Verification items for the finished model (mm, model axes). Face numbers are marked on the shaded views. A direction names the side the tool comes from. Round coordinates to 2 decimals unless told otherwise and drop trailing zeros. Loops run counter-clockwise (first coordinate to the right, second up) from the corner with the lowest first, then second, coordinate; pieces in that order, holes last. Notation, with made-up numbers: (-37.5, 6) - (-4.5, 6) arc R24 ccw to (-4.5, 34) - close; hole circle Ø10 at (50.5, 77.25). An arc over 180 degrees is marked (long way). Use a Markdown table: item, result. Add a question column.
```python
from build123d import *

# Parameters (mm, degrees)
F0_R           = 5.5
F1_DEPTH       = 60
F4_DEPTH       = 26
F4_DEPTH_BACK  = 26
F5_R           = 4
F6_DEPTH       = 5
F7_R           = 4.25
F8_DEPTH       = 15
F9_R           = 11
F10_DEPTH      = 25
F10_DEPTH_BACK = 25


# Not quite as in the source:
# - a feature names something its author has since deleted; it is built from what else it names


with BuildPart() as f1:
    # F0 (on Front) → F1 (new body)
    with BuildSketch(Plane.XZ):
        with BuildLine():
            ThreePointArc((-0.0872969156, -53.4805140133), (-11.9999962709, -41.4659778258), (-0.0575900904, -29.4809696761))
            Line((-0.0575900904, -29.4809696761), (-5.4639e-06, 17.0404876904))
            Line((-5.4639e-06, 17.0404876904), (-70.0428405992, 17.0404876904))
            Line((-70.0428405992, 17.0404876904), (-70.0428405992, 7.0404876904))
            Line((-70.0428405992, 7.0404876904), (-20.0428405992, 7.0404876904))
            Line((-20.0428405992, 7.0404876904), (-20.6929361639, -127.9595123096))
            Line((-20.6929361639, -127.9595123096), (-70.6929361639, -127.9595123096))
            Line((-70.6929361639, -127.9595123096), (-70.6929361639, -137.9595123096))
            Line((-70.6929361639, -137.9595123096), (-0.1918656855, -137.9595123096))
            Line((-0.1918656855, -137.9595123096), (-0.1862936956, -133.4580141387))
            ThreePointArc((-0.1862936956, -133.4580141387), (-11.9988136294, -121.4446249335), (-0.1565894029, -109.4605157571))
            Line((-0.1565894029, -109.4605157571), (-0.0872969156, -53.4805140133))
        make_face()
        with Locations((-5.947382655, -81.4808309078)):
            Circle(F0_R, mode=Mode.SUBTRACT)
    extrude(amount=F1_DEPTH)


with BuildPart() as f1_1:
    # F2: moved
    add(f1.part.moved(Location((0, 30, 0))))

    # F3 (on Front) → F4 (cut, two sides)
    with BuildSketch(Plane.XZ) as f4_sk:
        with BuildLine():
            ThreePointArc((0, -55.5154254436), (-14, -41.5154254436), (0, -27.5154254436))
            Line((0, -27.5154254436), (0, -26.5154254436))
            ThreePointArc((0, -26.5154254436), (-15, -41.5154254436), (0, -56.5154254436))
            Line((0, -56.5154254436), (0, -55.5154254436))
        make_face()
        with BuildLine():
            Line((0, -107.5154236555), (0, -106.5154236555))
            ThreePointArc((0, -106.5154236555), (-15, -121.5154236555), (0, -136.5154236555))
            Line((0, -136.5154236555), (0, -135.5154236555))
            ThreePointArc((0, -135.5154236555), (-14, -121.5154236555), (0, -107.5154236555))
        make_face()
    extrude(amount=F4_DEPTH, mode=Mode.SUBTRACT)
    extrude(f4_sk.sketch, amount=-F4_DEPTH_BACK, mode=Mode.SUBTRACT)

    # F5 (on face) → F6 (cut)
    with BuildSketch(Plane.XY.offset(-127.9595123096)):
        with Locations((-40.0428405992, -20)):
            Circle(F5_R)
        with Locations((-40.0428405992, 20)):
            Circle(F5_R)
    extrude(amount=-F6_DEPTH, mode=Mode.SUBTRACT)

    # F7 (on face) → F8 (cut)
    with BuildSketch(Plane.XY.offset(17.0404876904)):
        with Locations((-40.0428405992, 20)):
            Circle(F7_R)
        with Locations((-40.2286797762, -20)):
            Circle(F7_R)
    extrude(amount=-F8_DEPTH, mode=Mode.SUBTRACT)

    # F9 (on face) → F10 (cut, two sides)
    with BuildSketch(Plane.XY.offset(17.0404876904)) as f10_sk:
        with Locations((-40.1357601877, 0)):
            Circle(F9_R)
    extrude(amount=-F10_DEPTH, mode=Mode.SUBTRACT)
    extrude(f10_sk.sketch, amount=F10_DEPTH_BACK, mode=Mode.SUBTRACT)


solid = f1_1.part
```
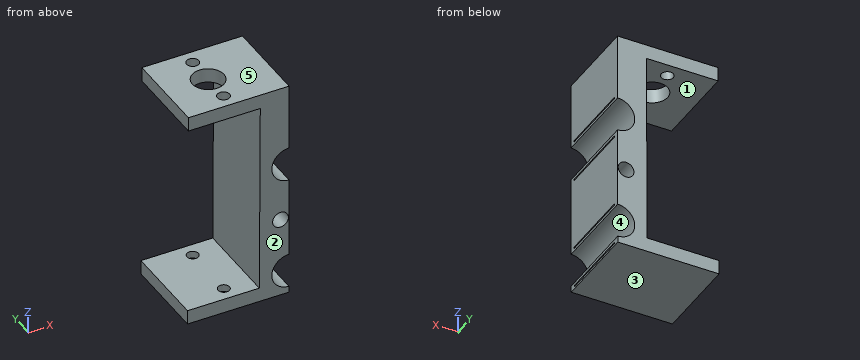
Q1. Section check B-B on x = -57.5. Record the cut outline in (y, z).
Q2. Section check D-D on y = 9. Record the cut outline in (x, z).
Q3. Go/stop test with flat-tipped pins: pin 1 Ø4 at (x, y) = (-38.5, -20.5) entering from +Z; pin 2 Ø8 at (y, z) = (-15, -82.5) entering from -X; pin 3 Ø6.5 at (x, y) = (-42, 19) entering from +Z; pin 4 Ø2 at (y, z) = (-8, -110) entering from -X. Record where each tip stops, or that it passes through.
Q4. Set-up check for the marked faces 1 and 2: record each of +Z, -Z, +X, -X, +Y, -Y from which the full face is reachable in a straight line by a thin tool's end or side.
Q5. Thickness scan on line 1 along Z through (x, y) = (-21, -18.5); line 2 along X through (y, z) = (24.5, -43); line 3 along X through (y, z) = (-13.5, -82). Record the ranges inside material, lowest first.
Q6. Release check for a two-part mould opening along Z. For the marked faces 3, 4 and 5 record: +Z half, -Z half, draft (parallel to the pull), parting line (faces both ways), or undercut.
Q7. Section check A-A on y = 20. State how many separate pieces and enclosed holes the cut face has, plus the area to 4 significant figures.
Q8. Section check C-C on z = -121. Record the cut outline in (x, y), plus the area to 3 significant figures.
Determined:
| question | item | result |
|---|---|---|
| 1 | outline | (-30, -137.96) - (30, -137.96) - (30, -127.96) - (-30, -127.96) - close; (-30, 7.04) - (30, 7.04) - (30, 17.04) - (-30, 17.04) - close |
| 2 | outline | (-70.69, -137.96) - (-0.19, -137.96) - (-0.19, -136.51) arc R15 cw to (-0.15, -106.52) - (-0.09, -56.52) arc R15 cw to (-0.05, -26.52) - (0, 17.04) - (-33.81, 17.04) - (-33.81, 7.04) - (-20.04, 7.04) - (-20.69, -127.96) - (-70.69, -127.96) - close; (-70.04, 7.04) - (-46.46, 7.04) - (-46.46, 17.04) - (-70.04, 17.04) - close; (-0.19, -135.51) - (-0.19, -133.46) arc R12 cw to (-0.16, -109.46) - (-0.15, -107.52) arc R14 ccw to start; (-0.09, -55.52) - (-0.09, -53.48) arc R12 cw to (-0.06, -29.48) - (-0.06, -27.52) arc R14 ccw to start; hole circle Ø11 at (-5.95, -81.48) |
| 3 | pin 1 | stops at z = -132.96 |
| 3 | pin 2 | stops at x = -20.49 |
| 3 | pin 3 | stops at z = 17.04 |
| 3 | pin 4 | stops at x = -20.61 |
| 4 | face 1 | -X, +Y, -Y |
| 4 | face 2 | +Z, -Z, +X, -X, -Y |
| 5 | line 1 | z = -137.96 to -127.96, 7.04 to 17.04 |
| 5 | line 2 | x = -20.28 to -14.93, -13.92 to -11.9 |
| 5 | line 3 | x = -20.47 to -11.42, -0.47 to -0.12 |
| 6 | face 3 | -Z half |
| 6 | face 4 | undercut |
| 6 | face 5 | +Z half |
| 7 | separate pieces | 4 |
| 7 | enclosed holes | 1 |
| 7 | area | 3,385 mm² |
| 8 | outline | (-20.66, -30) - (-11.99, -30) - (-11.99, 30) - (-20.66, 30) - close; hole (-14.99, -26) - (-13.99, -26) - (-13.99, 26) - (-14.99, 26) - close |
| 8 | area | 468 mm² |
